```python
from build123d import *

# Parameters (mm, degrees)
F0_W     = 25
F0_H     = 40
F0_R     = 3
F1_DEPTH = 6
F2_W     = 6
F2_H     = 40
F3_DEPTH = 120
F4_R     = 12.5
F5_DEPTH = 25.4
F6_W     = 6
F6_H     = 15
F7_DEPTH = 15
F8_R     = 1.5
F9_DEPTH = 20.001


with BuildPart() as f1:
    # F0 (on Front) → F1 (new body)
    with BuildSketch(Plane.XZ):
        Rectangle(F0_W, F0_H)
        with Locations((-3, -14)):
            Circle(F0_R, mode=Mode.SUBTRACT)
        with Locations((-3, 14)):
            Circle(F0_R, mode=Mode.SUBTRACT)
    extrude(amount=F1_DEPTH)

    # F2 (on face) → F3 (join)
    with BuildSketch(Plane.XZ.offset(6)):
        with Locations((9.5, 0)):
            Rectangle(F2_W, F2_H)
    extrude(amount=F3_DEPTH)

    # F4 (on face) → F5 (cut)
    with BuildSketch(Plane(origin=(6.5, 0, 0), x_dir=(0, -1, 0), z_dir=(-1, 0, 0))):
        Polygon((126, 20), (6, 20), (126, 15), align=None)
        Polygon((126, -15), (6, -20), (126, -20), align=None)
        with Locations((101.661727, 0)):
            Circle(F4_R)
        with Locations((73.966578, 0)):
            Circle(F4_R)
        with Locations((48.03938, 0)):
            Circle(F4_R)
        with Locations((22.46337, 0)):
            Circle(F4_R)
    extrude(amount=-F5_DEPTH, mode=Mode.SUBTRACT)

    # F6 (on face) → F7 (join)
    with BuildSketch(Plane.XZ.offset(126)):
        with Locations((9.5, -7.5)):
            Rectangle(F6_W, F6_H)
    extrude(amount=F7_DEPTH)

    # F8 (on face) → F9 (cut, through all)
    with BuildSketch(Plane.XY):
        with Locations((9.5, -135)):
            Circle(F8_R)
    extrude(amount=-F9_DEPTH, mode=Mode.SUBTRACT)


solid = f1.part
```
Design review of the part built by this model. Coordinates are the model's own, in mm. A direction names the side the tool comes from. Give positions to 0.01 mm unless a question says otherwise; leave off trailing zeros. Write each loop counter-clockwise with the first axis right and the second up, starting at its lowest first coordinate (ties: lowest second). Pieces come first, ordered by that corner, then holes. Notation, with made-up numbers: (75.5, 5) - (112.5, 5) arc R30 ccw to (112.5, 38) - close; hole circle Ø7 at (-33, 43). An arc over 180 degrees is marked (long way). Return JSON: item names as keys, results as strings. Group by question number.
(1) We need section C-C, the plane x = -3. Give the boundary of the cut face in (y, z).
(2) We need section D-D, the plane z = -3.5. Give the boundary of the cut face in (x, y).
(3) We need section B-B, the plane y = -135. Give the boundary of the cut face in (x, z).
(4) We need section A-A, the plane x = 9.5. Give the boundary of the cut face in (y, z), then the cut area to 3 significant figures.
(5) Machinability: for faces 4 (the flat face through (9, -133, 0)), 5 (the flat face through (0, 0, 0)), 6 (the flat face through (6.5, -73, -14)), 7 (the flat face through (9, -133, -15)), which of the approach directions +Z, -Z, +X, -X, +Y, -Y give a long, thin tool a straight path to every point of the face, cutting with its end or side? Answer none if there is none.
(6) Insertion check: pin 1 (5 mm diameter, centred on x = 9, y = -131, fed in from +Z); pin 2 (6.5 mm diameter, centred on x = 8.5, y = -137, fed in from -Z); pin 3 (9.5 mm diameter, centred on x = -3, z = -14, fed in from -Y). Each pin has a flat end and moves straight along its axis. Give the tip position at first contact, or say it passes through.
(7) To check wall thickness, follow probe 1 along Z at (x, y) = (-3, -3.75); probe 2 along Y at (x, z) = (9.5, -7.25); probe 3 along X at (y, z) = (-135, -4). State the ranges of each line that lie inside material, in increasing order.
(8) Mouldability with a two-part tool opening along Z and no side actions: class faces 1 (the flat face through (0, -3, 20)), 2 (the flat face through (9, -126, 8)), 3 (the cylindrical face through (9.458, -34.386, 3.755)) as +Z half, -Z half, draft (parallel to the pull), parting line (faces both ways), or undercut.
Reported:
{
 "1": {"outline": "(-6, -20) - (0, -20) - (0, -17) - (-6, -17) - close; (-6, -11) - (0, -11) - (0, 11) - (-6, 11) - close; (-6, 17) - (0, 17) - (0, 20) - (-6, 20) - close"},
 "2": {"outline": "(-12.5, -6) - (6.5, -6) - (6.5, -10.46) - (12.5, -10.46) - (12.5, 0) - (-12.5, 0) - close; (6.5, -141) - (12.5, -141) - (12.5, -113.66) - (6.5, -113.66) - close; (6.5, -89.66) - (12.5, -89.66) - (12.5, -85.97) - (6.5, -85.97) - close; (6.5, -61.97) - (12.5, -61.97) - (12.5, -60.04) - (6.5, -60.04) - close; (6.5, -36.04) - (12.5, -36.04) - (12.5, -34.46) - (6.5, -34.46) - close; hole circle Ø3 at (9.5, -135)"},
 "3": {"outline": "(6.5, -15) - (8, -15) - (8, 0) - (6.5, 0) - close; (11, -15) - (12.5, -15) - (12.5, 0) - (11, 0) - close"},
 "4": {"outline": "(-141, -15) - (-136.5, -15) - (-136.5, 0) - (-141, 0) - close; (-133.5, -15) - (-126, -15) - (-6, -20) - (0, -20) - (0, 20) - (-6, 20) - (-126, 15) - (-126, 0) - (-133.5, 0) - close; hole circle Ø25 at (-101.66, 0); hole circle Ø25 at (-73.97, 0); hole circle Ø25 at (-48.04, 0); hole circle Ø25 at (-22.46, 0)", "area": "2,660 mm2"},
 "5": {"face 4": "+Z, +X, -X, -Y", "face 5": "+Z, -Z, +X, -X, +Y", "face 6": "+Z, -Z, -X, -Y", "face 7": "-Z, +X, -X, -Y"},
 "6": {"pin 1": "stops at z = 0", "pin 2": "stops at z = -15", "pin 3": "stops at y = -6"},
 "7": {"probe 1": "z = -20 to -17, -11 to 11, 17 to 20", "probe 2": "y = -141 to -136.5, -133.5 to -111.84, -91.48 to -84.15, -63.78 to -58.22, -37.86 to -32.65, -12.28 to 0", "probe 3": "x = 6.5 to 8, 11 to 12.5"},
 "8": {"face 1": "+Z half", "face 2": "draft", "face 3": "undercut"}
}
